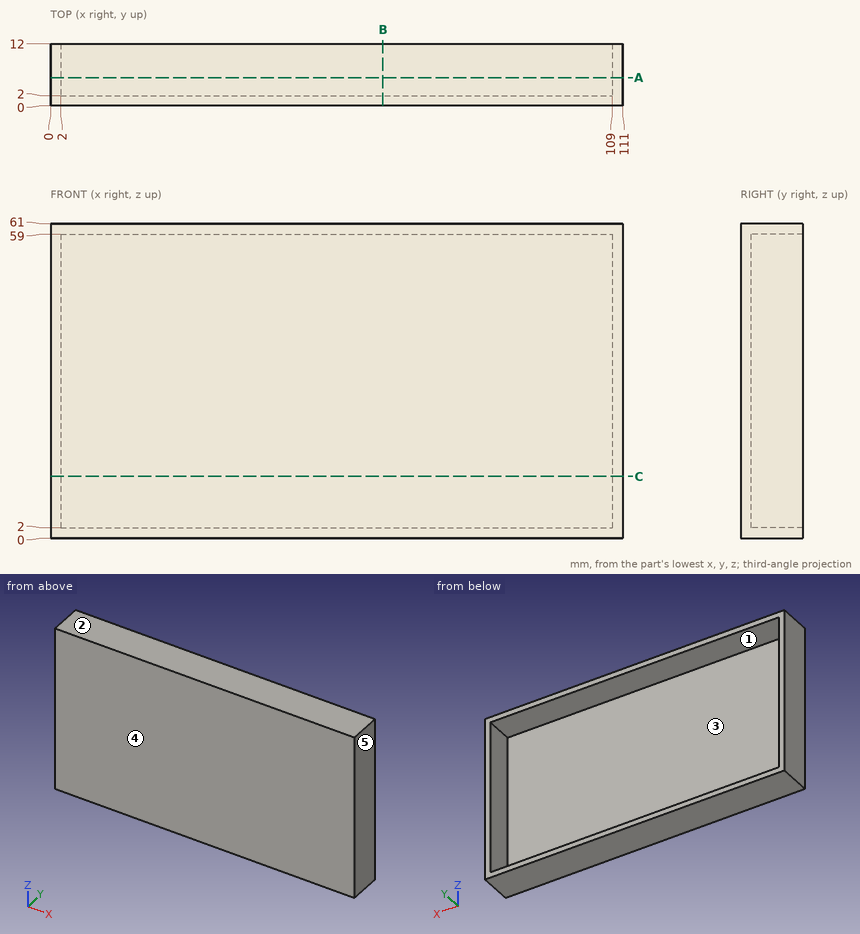
Job drawing, mm, ordinate dimensions from the low corner. One solid piece. A direction names the side the tool comes from. Coordinates: 2 decimals unless noted, no trailing zeros. Order: outer loops, then holes, each group sorted by start corner. A loop starts at its lowest first (then second) coordinate and runs counter-clockwise, first axis right, second up. Notation, with made-up numbers: (2, -37) -> (18, -37) arc R20 ccw to (18, -2) -> close; hole circle Ø4 at (42, 29.5). An arc over 180 degrees is marked (long way). Answer in a Markdown table with one row per item. Add a question column.
Q1. Which spindle directions (+Z, -Z, +X, -X, +Y, -Y) get a long thin tool onto all of the face, cutting with end or side? Do the marked faces 1 and 2. Say none if no direction does.
Q2. Mould opens along X. For the marked faces 3, 4 and 5 say: +X half, -X half, draft (parallel to the pull), parting line (faces both ways), or undercut.
Q3. Band-saw the part on C-C, the plane z = 12. List the corners of the cut face in (x, y).
Q4. Wall check: line 1 along X through (y, z) = (7, 29.5); line 2 along Z through (x, y) = (44.5, 9.5); line 3 along Y through (x, z) = (59.5, 12.5). Give the ranges that are in metal, low to high. Write a range as [from, to].
Q5. Band-saw the part on A-A, the plane y = 5.5. List the corners of the cut face in (x, z).
Q6. Drop a flat-ended pin along its axis: pin 1 (8 mm diameter, centred on x = 77, z = 46, fed in from -Y). Give the stop position or say it passes through.
Q7. Band-saw the part on B-B, the plane x = 64.5. List the corners of the cut face in (y, z).
Answers follow:
| question | item | result |
|---|---|---|
| 1 | face 1 | +Y |
| 1 | face 2 | +Z, +X, -X, +Y, -Y |
| 2 | face 3 | undercut |
| 2 | face 4 | draft |
| 2 | face 5 | +X half |
| 3 | outline | (0, 0) -> (111, 0) -> (111, 12) -> (109, 12) -> (109, 2) -> (2, 2) -> (2, 12) -> (0, 12) -> close |
| 4 | line 1 | [0, 2], [109, 111] |
| 4 | line 2 | [0, 2], [59, 61] |
| 4 | line 3 | [0, 2] |
| 5 | outline | (0, 0) -> (111, 0) -> (111, 61) -> (0, 61) -> close; hole (2, 2) -> (109, 2) -> (109, 59) -> (2, 59) -> close |
| 6 | pin 1 | y = 0 |
| 7 | outline | (0, 0) -> (12, 0) -> (12, 2) -> (2, 2) -> (2, 59) -> (12, 59) -> (12, 61) -> (0, 61) -> close |
